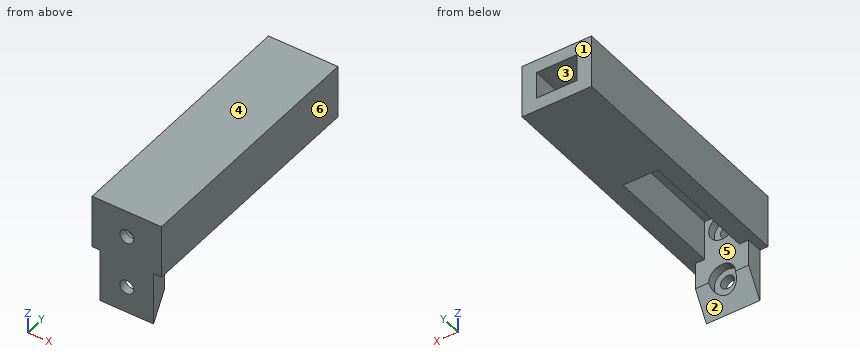
from build123d import *

# Parameters (mm, degrees)
EXTRUDE_1_DEPTH      = 6
SKETCH_2_R           = 2.6
CUT_EXTRUDE_1_DEPTH  = 6
SKETCH_3_R           = 5
CUT_EXTRUDE_2_DEPTH  = 3
SKETCH_4_W           = 26
SKETCH_4_H           = 20
SKETCH_4_W_2         = 15
SKETCH_4_H_2         = 10
EXTRUDE_2_DEPTH      = 89
CUT_EXTRUDE_5_DEPTH  = 5
SKETCH_6_W           = 1
SKETCH_6_H           = 44
EXTRUDE_3_DEPTH      = 15
SKETCH_8_W           = 26
SKETCH_8_H           = 20
SKETCH_8_R           = 2.6
EXTRUDE_4_DEPTH      = 6
SKETCH_9_R           = 5
CUT_EXTRUDE_6_DEPTH  = 3
CUT_EXTRUDE_7_DEPTH  = 30
SKETCH_11_W          = 3
SKETCH_11_H          = 6
CUT_EXTRUDE_8_DEPTH  = 30
CUT_EXTRUDE_10_DEPTH = 45


with BuildPart() as part:
    # 草图1 → 凸台-拉伸1 (new body)
    with BuildSketch(Plane(origin=(0, 0, 0), x_dir=(1, 0, 0), z_dir=(0, 1, 0))):
        Polygon((-10, -10), (10, -10), (13, -10), (13, 10), (10, 10), (-10, 10), (-13, 10), (-13, -10), align=None)
    extrude(amount=EXTRUDE_1_DEPTH)

    # 草图2 → 切除-拉伸1 (cut)
    with BuildSketch(Plane(origin=(0, 6, 0), x_dir=(1, 0, 0), z_dir=(0, 1, 0))):
        with Locations(Location((0, 0, 0), (0, 0, 270))):
            Circle(SKETCH_2_R)
    extrude(amount=-CUT_EXTRUDE_1_DEPTH, mode=Mode.SUBTRACT)

    # 草图3 → 切除-拉伸2 (cut)
    with BuildSketch(Plane(origin=(0, 6, 0), x_dir=(1, 0, 0), z_dir=(0, 1, 0))):
        with Locations(Location((0, 0, 0), (0, 0, 270))):
            Circle(SKETCH_3_R)
    extrude(amount=-CUT_EXTRUDE_2_DEPTH, mode=Mode.SUBTRACT)

    # 草图4 → 凸台-拉伸2 (add)
    with BuildSketch(Plane(origin=(0, 6, 0), x_dir=(1, 0, 0), z_dir=(0, 1, 0))):
        Rectangle(SKETCH_4_W, SKETCH_4_H)
        Rectangle(SKETCH_4_W_2, SKETCH_4_H_2, mode=Mode.SUBTRACT)
    extrude(amount=EXTRUDE_2_DEPTH)

    # 草图5 → 切除-拉伸5 (cut)
    with BuildSketch(Plane(origin=(0, 0, -10), x_dir=(-1, 0, 0), z_dir=(0, 0, -1))):
        Polygon((0, 6), (7.5, 6), (7.5, 15), (7.5, 30), (7.5, 50), (-7.5, 50), (-7.5, 30), (-7.5, 15), (-7.5, 6), align=None)
    extrude(amount=-CUT_EXTRUDE_5_DEPTH, mode=Mode.SUBTRACT)

    # 草图6 → 凸台-拉伸3 (add)
    with BuildSketch(Plane(origin=(0, 0, -10), x_dir=(-1, 0, 0), z_dir=(0, 0, -1))):
        with Locations((7, 28)):
            Rectangle(SKETCH_6_W, SKETCH_6_H)
        with Locations((-7, 28)):
            Rectangle(SKETCH_6_W, SKETCH_6_H)
    extrude(amount=-EXTRUDE_3_DEPTH)

    # 草图8 → 凸台-拉伸4 (add)
    with BuildSketch(Plane.XZ):
        with Locations((0, -20)):
            Rectangle(SKETCH_8_W, SKETCH_8_H)
        with Locations(Location((0, -20, 0), (0, 0, 270))):
            Circle(SKETCH_8_R, mode=Mode.SUBTRACT)
    extrude(amount=-EXTRUDE_4_DEPTH)

    # 草图9 → 切除-拉伸6 (cut)
    with BuildSketch(Plane(origin=(0, 6, 0), x_dir=(1, 0, 0), z_dir=(0, 1, 0))):
        with Locations(Location((0, 20, 0), (0, 0, 270))):
            Circle(SKETCH_9_R)
    extrude(amount=-CUT_EXTRUDE_6_DEPTH, mode=Mode.SUBTRACT)

    # 草图10 → 切除-拉伸7 (cut)
    with BuildSketch(Plane.ZY.offset(13)):
        Polygon((-20, 6), (-30, 0), (-30, 6), align=None)
    extrude(amount=-CUT_EXTRUDE_7_DEPTH, mode=Mode.SUBTRACT)

    # 草图11 → 切除-拉伸8 (cut)
    with BuildSketch(Plane(origin=(0, 0, -10), x_dir=(-1, 0, 0), z_dir=(0, 0, -1))):
        with Locations((-11.5, 3)):
            Rectangle(SKETCH_11_W, SKETCH_11_H)
        with Locations((11.5, 3)):
            Rectangle(SKETCH_11_W, SKETCH_11_H)
    extrude(amount=CUT_EXTRUDE_8_DEPTH, mode=Mode.SUBTRACT)

    # 草图12 → 切除-拉伸10 (cut)
    with BuildSketch(Plane(origin=(0, 95, 0), x_dir=(1, 0, 0), z_dir=(0, 1, 0))):
        Polygon((-7.5, 5.1), (-7.5, 5), (7.5, 5), (7.5, -5), (7.6, -5), (7.6, 5.1), align=None)
        Polygon((-7.6, -5.1), (-7.6, 5.1), (-7.5, 5.1), (-7.5, 5), (-7.5, -5), (7.5, -5), (7.6, -5), (7.6, -5.1), align=None)
    extrude(amount=-CUT_EXTRUDE_10_DEPTH, mode=Mode.SUBTRACT)


solid = part.part
The model under review builds one solid part; all positions refer to its coordinate system, in mm. Face numbers are marked on the shaded views. A direction names the side the tool comes from. Give positions to 0.01 mm unless a question says otherwise; leave off trailing zeros. Loops run counter-clockwise (first coordinate to the right, second up) from the corner with the lowest first, then second, coordinate; pieces in that order, holes last. Notation, with made-up numbers: (38, -32) -> (47, -32) arc R34 ccw to (47, 1) -> close; hole circle Ø6 at (31.25, 15). An arc over 180 degrees is marked (long way). Put each result on its own line as item: value. Start each with the question number.
1. Wall thickness on probe 1 along Z at (x, y) = (0, 5); probe 2 along Z at (x, y) = (-5, 72.5); probe 3 along X at (y, z) = (2.15, 0): over which ranges is each line inside the solid? List them lowest first.
2. We need section A-A on z = 0. State the section outline as (x, y) points.
3. For the marked faces 5 and 6, list the 3-axis set-ups (+Z, -Z, +X, -X, +Y, -Y) from which the entire face can be reached by the end or side of a thin tool; tool diameter is ignored.
4. Clearance check with flat-ended pins moving along their axes: P1, Ø4.5, axis at x = -0.5, y = 81.5, coming from the -Z side; P2, Ø5, axis at y = 3.5, z = -24.5, coming from the -X side; P3, Ø4, axis at x = -1.5, y = 26, coming from the -Z side. State where each tip first meets the part, or that it passes through.
5. We need section D-D on z = -7.5. State the section outline as (x, y) points.
6. Mouldability with a two-part tool opening along Z and no side actions: class the marked faces 1, 2, 3 and 4 as released by +Z, released by -Z, zero draft, split by the parting line, or undercut.
7. We need section C-C on y = 84. State the section outline as (x, z) points.
8. We need section B-B on x = -4. State the section outline as (y, z) points, then the cut area to 3 significant figures.
Determined:
1. probe 1: -15 to -5, 5 to 10
1. probe 2: -10 to -5.1, 5.1 to 10
1. probe 3: -13 to -2.6, 2.6 to 13
2. outline: (-13, 0) -> (-2.6, 0) -> (-2.6, 3) -> (-5, 3) -> (-5, 6) -> (-6.5, 6) -> (-6.5, 50) -> (-7.6, 50) -> (-7.6, 95) -> (-13, 95) -> close; (2.6, 0) -> (13, 0) -> (13, 95) -> (7.6, 95) -> (7.6, 50) -> (6.5, 50) -> (6.5, 6) -> (5, 6) -> (5, 3) -> (2.6, 3) -> close
3. face 5: -Z
3. face 6: +Z, -Z, +X, +Y, -Y
4. P1: z = -10
4. P2: x = -10
4. P3: z = 5
5. outline: (-13, 0) -> (13, 0) -> (13, 95) -> (-13, 95) -> close; hole (-6.5, 6) -> (6.5, 6) -> (6.5, 50) -> (-6.5, 50) -> close
6. face 1: zero draft
6. face 2: released by -Z
6. face 3: undercut
6. face 4: released by +Z
7. outline: (-13, -10) -> (13, -10) -> (13, 10) -> (-13, 10) -> close; hole (-7.6, -5.1) -> (7.6, -5.1) -> (7.6, 5.1) -> (-7.6, 5.1) -> close
8. outline: (0, -30) -> (4.2, -23) -> (3, -23) -> (3, -17) -> (6, -17) -> (6, -3) -> (3, -3) -> (3, 3) -> (6, 3) -> (6, 5) -> (50, 5) -> (50, 5.1) -> (95, 5.1) -> (95, 10) -> (0, 10) -> close; (50, -10) -> (95, -10) -> (95, -5.1) -> (50, -5.1) -> close
8. area: 838 mm^2
